from build123d import *

# Parameters (mm, degrees)
F0_R     = 4
F1_DEPTH = 38
F2_R     = 13
F2_R_2   = 4
F3_DEPTH = 12
F4_R     = 25.5
F4_R_2   = 13
F5_DEPTH = 71
F6_R     = 13
F7_DEPTH = 7


with BuildPart() as f1:
    # F0 (on Top) → F1 (new body)
    with BuildSketch(Plane.XY):
        Circle(F0_R)
    extrude(amount=F1_DEPTH)

    # F2 (on face) → F3 (join)
    with BuildSketch(Plane.XY.offset(38)):
        Circle(F2_R)
        Circle(F2_R_2, mode=Mode.SUBTRACT)
        Circle(F2_R_2)
    extrude(amount=F3_DEPTH)

    # F4 (on face) → F5 (join)
    with BuildSketch(Plane.XY.offset(50)):
        Circle(F4_R)
        Circle(F4_R_2, mode=Mode.SUBTRACT)
        Circle(F4_R_2)
    extrude(amount=F5_DEPTH)

    # F6 (on face) → F7 (join)
    with BuildSketch(Plane.XY.offset(121)):
        Circle(F6_R)
    extrude(amount=F7_DEPTH)


solid = f1.part
The model under review builds one solid part; all positions refer to its coordinate system, in mm. A direction names the side the tool comes from. Round coordinates to 2 decimals unless told otherwise and drop trailing zeros. Write each loop counter-clockwise with the first axis right and the second up, starting at its lowest first coordinate (ties: lowest second). Pieces come first, ordered by that corner, then holes. Notation, with made-up numbers: (-30, -17) - (3, -17) arc R25 cw to (3, 7) - close; hole circle Ø4 at (-11.5, -3.5). An arc over 180 degrees is marked (long way). One line per item, written item: value. Start each with the question number.
1. Consider section D-D on y = -9.5. Write out the cut boundary in (x, z).
2. Consider section A-A on y = 0. Write out the cut boundary in (x, z), and give its area (3 significant figures).
3. Clearance check with flat-ended pins moving along their axes: P1, Ø12, axis at x = -16, y = -19.5, coming from the +Z side; P2, Ø10, axis at x = 20.5, z = 73, coming from the -Y side; P3, Ø12, axis at y = -13, z = 96, coming from the -X side; P4, Ø8, axis at y = -8.5, z = 17.5, coming from the +X side. State where each tip first meets the part, or that it passes through.
4. Machinability: for faces 1 (the face through (-12, 6, 121)), 2 (the face through (3, 3, 38)), 3 (the face through (0, 0, 128)), which of the approach directions +Z, -Z, +X, -X, +Y, -Y give a long, thin tool a straight path to every point of the face, cutting with its end or side? Answer none if there is none.
5. To check wall thickness, follow L1, parallel to Z at x = 5.5, y = -22; L2, parallel to Z at x = -8.5, y = 5; L3, parallel to Y at x = 11, z = 96. State the ranges of each line that lie inside material, in increasing order. Write a range as from..to.
6. Consider section C-C on z = 78. Write out the cut boundary in (x, y).
Checks:
1. outline: (-23.66, 50) - (-8.87, 50) - (-8.87, 38) - (8.87, 38) - (8.87, 50) - (23.66, 50) - (23.66, 121) - (8.87, 121) - (8.87, 128) - (-8.87, 128) - (-8.87, 121) - (-23.66, 121) - close
2. outline: (-25.5, 50) - (-13, 50) - (-13, 38) - (-4, 38) - (-4, 0) - (4, 0) - (4, 38) - (13, 38) - (13, 50) - (25.5, 50) - (25.5, 121) - (13, 121) - (13, 128) - (-13, 128) - (-13, 121) - (-25.5, 121) - close
2. area: 4,420 mm^2
3. P1: stops at z = 121
3. P2: stops at y = -20.25
3. P3: stops at x = -24.52
3. P4: passes through
4. face 1: +Z
4. face 2: -Z
4. face 3: +Z, +X, -X, +Y, -Y
5. L1: z = 50..121
5. L2: z = 38..128
5. L3: y = -23.01..23.01
6. outline: circle Ø51 at (0, 0)
